Part model, mm, in its own coordinate system. A direction names the side the tool comes from. Round coordinates to 2 decimals unless told otherwise and drop trailing zeros. Loops run counter-clockwise (first coordinate to the right, second up) from the corner with the lowest first, then second, coordinate; pieces in that order, holes last. Notation, with made-up numbers: (-11, 71.25) -> (38, 71.25) arc R35 cw to (38, 108.25) -> close; hole circle Ø8 at (70.5, 6). An arc over 180 degrees is marked (long way). Use a Markdown table: item, result. Add a question column.
Item 1: Flat gauge pins, fed straight in: pin 1 (11 mm diameter, centred on x = 62.875, z = 30, fed in from +Y); pin 2 (3.5 mm diameter, centred on x = 62.875, z = 10, fed in from +Y) (1 decimal). Where does each tip first touch, or does it go through?
Item 2: Cut at B-B, the plane z = 22. List the corners of the cut face in (x, y) (3 decimals), plus the area to 3 significant figures.
Item 3: Cut at A-A, the plane y = 2. List the corners of the cut face in (x, z) (3 decimals), plus the area to 3 significant figures.
Item 4: Two-plate mould, pull along Y, no slides. Class faces 1 (the face through (-62, 16.42, 27)), 2 (the face through (-65.64, 11.83, 30.87)), 3 (the face through (63, 7.375, 20)): pulls with the +Y half, pulls with the -Y half, needs draft (parallel to the pull), parting line crosses it, or undercut.
Item 5: Which spindle directions (+Z, -Z, +X, -X, +Y, -Y) get a long thin tool onto all of the face, cutting with end or side? Do faces 4 (the face through (-68.99, 18.24, 9.73)), 5 (the face through (-63, -7.375, 20)), 6 (the face through (64.43, 11.83, 7.55)). Say none if no direction does.
Item 6: Probe line 1 (X direction, y = -6, z = 4) (3 decimals); line 2 (Z direction, x = 62.5, y = 18.5); line 3 (X direction, y = 11.5, z = 10) (3 decimals). List the from-to ranges inside material, lowest first. Write a range as [from, to].
Item 7: Cut at C-C, the plane z = 30. State how many separate pieces and enclosed holes the cut face has, plus the area to 3 significant figures.
```python
from build123d import *

# Parameters (mm, degrees)
SKETCH2_W                               = 171.25
SKETCH2_H                               = 40
BOSS_EXTRUDE1_DEPTH                     = 40
SKETCH3_W                               = 20.25
SKETCH3_H                               = 14.75
CUT_EXTRUDE1_DEPTH                      = 97.600417313
CHAMFER1_SIZE                           = 5
FILLET1_R                               = 2.5
CBORE_FOR_M5_HEX_HEAD_BOLT1_D           = 5.8
CBORE_FOR_M5_HEX_HEAD_BOLT1_CBORE_D     = 12.24
CBORE_FOR_M5_HEX_HEAD_BOLT1_CBORE_DEPTH = 3.58
MIRROR2_COPY_1_D                        = 5.8
MIRROR2_COPY_1_CBORE_D                  = 12.24
MIRROR2_COPY_1_CBORE_DEPTH              = 3.58


with BuildPart() as part:
    # Sketch2 → Boss-Extrude1 (new body)
    with BuildSketch(Plane.XY):
        Rectangle(SKETCH2_W, SKETCH2_H)
    extrude(amount=BOSS_EXTRUDE1_DEPTH)

    # Sketch3 → Cut-Extrude1 (cut, through all)
    with BuildSketch(Plane.XY.offset(40)):
        with Locations((-62.875, 0)):
            Rectangle(SKETCH3_W, SKETCH3_H)
        with Locations((62.875, 0)):
            Rectangle(SKETCH3_W, SKETCH3_H)
    extrude(amount=-CUT_EXTRUDE1_DEPTH, mode=Mode.SUBTRACT)

    # Chamfer1
    chamfer1_edges = [part.edges().sort_by_distance(p)[0] for p in [
        (85.625, -20, 20),
        (-85.625, -20, 20),
        (-85.625, 20, 20),
        (85.625, 20, 20),
    ]]
    chamfer(chamfer1_edges, length=CHAMFER1_SIZE)

    # Fillet1
    fillet1_edges = [part.edges().sort_by_distance(p)[0] for p in [
        (-80.625, 20, 20),
        (80.625, 20, 20),
        (85.625, -15, 20),
        (85.625, 15, 20),
        (-80.625, -20, 20),
        (80.625, -20, 20),
        (-85.625, 15, 20),
        (-85.625, -15, 20),
    ]]
    fillet(fillet1_edges, radius=FILLET1_R)

    # CBORE for M5 Hex Head Bolt1 (through all)
    with Locations(Plane(origin=(0, 20, 0), x_dir=(1, 0, 0), z_dir=(0, 1, 0))):
        with Locations((-62.875, -10)):
            cbore_for_m5_hex_head_bolt1 = CounterBoreHole(CBORE_FOR_M5_HEX_HEAD_BOLT1_D / 2, CBORE_FOR_M5_HEX_HEAD_BOLT1_CBORE_D / 2, CBORE_FOR_M5_HEX_HEAD_BOLT1_CBORE_DEPTH)

    # Mirror1: CBORE for M5 Hex Head Bolt1 across plane
    add(cbore_for_m5_hex_head_bolt1.mirror(Plane.XY.offset(20)), mode=Mode.SUBTRACT)

    # Mirror2: CBORE for M5 Hex Head Bolt1 across plane
    add(cbore_for_m5_hex_head_bolt1.mirror(Plane(origin=(0, 0, 0), x_dir=(0, 0, 1), z_dir=(1, 0, 0))), mode=Mode.SUBTRACT)

    # Mirror2 copy 1 (through all)
    with Locations(Plane(origin=(0, 20, 40), x_dir=(-1, 0, 0), z_dir=(0, 1, 0))):
        with Locations((-62.875, -10)):
            CounterBoreHole(MIRROR2_COPY_1_D / 2, MIRROR2_COPY_1_CBORE_D / 2, MIRROR2_COPY_1_CBORE_DEPTH)


solid = part.part
```
A:
| question | item | result |
|---|---|---|
| 1 | pin 1 | stops at y = 16.42 |
| 1 | pin 2 | passes through |
| 2 | outline | (-85.625, -13.964) arc R2.5 ccw to (-84.893, -15.732) -> (-81.357, -19.268) arc R2.5 ccw to (-79.589, -20) -> (79.589, -20) arc R2.5 ccw to (81.357, -19.268) -> (84.893, -15.732) arc R2.5 ccw to (85.625, -13.964) -> (85.625, 13.964) arc R2.5 ccw to (84.893, 15.732) -> (81.357, 19.268) arc R2.5 ccw to (79.589, 20) -> (-79.589, 20) arc R2.5 ccw to (-81.357, 19.268) -> (-84.893, 15.732) arc R2.5 ccw to (-85.625, 13.964) -> close; hole (-73, -7.375) -> (-52.75, -7.375) -> (-52.75, 7.375) -> (-73, 7.375) -> close; hole (52.75, -7.375) -> (73, -7.375) -> (73, 7.375) -> (52.75, 7.375) -> close |
| 2 | area | 6,200 mm^2 |
| 3 | outline | (-85.625, 0) -> (-73, 0) -> (-73, 40) -> (-85.625, 40) -> close; (-52.75, 0) -> (52.75, 0) -> (52.75, 40) -> (-52.75, 40) -> close; (73, 0) -> (85.625, 0) -> (85.625, 40) -> (73, 40) -> close |
| 3 | area | 5,230 mm^2 |
| 4 | face 1 | pulls with the +Y half |
| 4 | face 2 | needs draft |
| 4 | face 3 | undercut |
| 5 | face 4 | +Y |
| 5 | face 5 | +Z, -Z |
| 5 | face 6 | +Y, -Y |
| 6 | line 1 | x = [-85.625, -73], [-52.75, 52.75], [73, 85.625] |
| 6 | line 2 | z = [0, 3.89], [16.11, 23.89], [36.11, 40] |
| 6 | line 3 | x = [-85.625, -65.775], [-59.975, 59.975], [65.775, 85.625] |
| 7 | separate pieces | 3 |
| 7 | enclosed holes | 0 |
| 7 | area | 5,860 mm^2 |
